Source: CAD feature listing. Evaluate the final solid. Frame: model axes, mm. Round coordinates to 2 decimals unless told otherwise and drop trailing zeros. Order: outer loops, then holes, each group sorted by start corner. A loop starts at its lowest first (then second) coordinate and runs counter-clockwise, first axis right, second up. Notation, with made-up numbers: (-20.75, 45) -> (35.25, 45) arc R22 cw to (35.25, 61) -> close; hole circle Ø10 at (70.5, 63). An arc over 180 degrees is marked (long way). Answer as CSV lines item,"result".
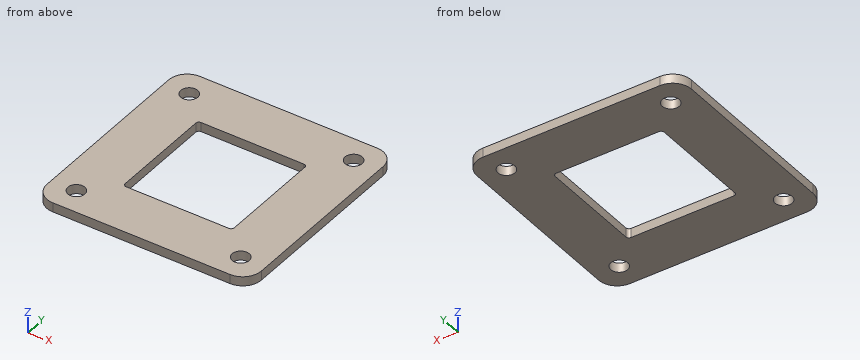
Autodesk Inventor part; units mm, degrees
ref_plane "YZ Plane" through (0, 0, 0) normal (1, 0, 0) x (0, 1, 0)
ref_plane "XZ Plane" through (0, 0, 0) normal (0, 1, 0) x (-1, 0, 0)
ref_plane "XY Plane" through (0, 0, 0) normal (0, 0, 1) x (1, 0, 0)
sketch "Sketch1" plane through (0, 0, 0) normal (0, 0, 1) x (1, 0, 0)
  line L0 (-34.6, -34.6) -> (34.6, -34.6)
  line L1 (34.6, -34.6) -> (34.6, 34.6)
  line L2 (34.6, 34.6) -> (-34.6, 34.6)
  line L3 (-34.6, 34.6) -> (-34.6, -34.6)
  line L4 (-34.6, -34.6) -> (34.6, 34.6) construction
  line L5 (34.6, -34.6) -> (-34.6, 34.6) construction
  line L6 (17.6, -17.6) -> (-17.6, -17.6)
  line L7 (-17.6, -17.6) -> (-17.6, 17.6)
  line L8 (-17.6, 17.6) -> (17.6, 17.6)
  line L9 (17.6, 17.6) -> (17.6, -17.6)
  line L10 (17.6, -17.6) -> (-17.6, 17.6) construction
  line L11 (-17.6, -17.6) -> (17.6, 17.6) construction
  point P0 (0, 0)
  dimension "d172" = 35.2
  dimension "d181" = 17
  dimension "d187" = 17
extrude "Plate5" add sketch "Sketch1" along normal blind 3
sketch "Sketch9" plane through (0, 0, 3) normal (0, 0, 1) x (1, 0, 0)
  circle A0 centre (26.5165, -26.5165) radius 2.75
  line L0 (26.5165, 26.5165) -> (-26.5165, 26.5165) construction
  line L1 (-26.5165, 26.5165) -> (-26.5165, -26.5165) construction
  line L2 (-26.5165, -26.5165) -> (26.5165, -26.5165) construction
  line L3 (26.5165, -26.5165) -> (26.5165, 26.5165) construction
  line L4 (26.5165, 26.5165) -> (-26.5165, -26.5165) construction
  line L5 (-26.5165, 26.5165) -> (26.5165, -26.5165) construction
  circle A1 centre (-26.5165, -26.5165) radius 2.75
  circle A2 centre (26.5165, 26.5165) radius 2.75
  circle A3 centre (-26.5165, 26.5165) radius 2.75
  circle A4 centre (0, 0) radius 37.5 construction
  line L6 (-17.6, -17.6) -> (-17.6, 17.6)
  line L7 (-17.6, 17.6) -> (17.6, 17.6)
  line L8 (17.6, 17.6) -> (17.6, -17.6)
  line L9 (17.6, -17.6) -> (-17.6, -17.6)
  line L10 (34.6, -34.6) -> (-34.6, -34.6)
  line L11 (34.6, 34.6) -> (34.6, -34.6)
  line L12 (-34.6, 34.6) -> (34.6, 34.6)
  line L13 (-34.6, -34.6) -> (-34.6, 34.6)
  line L14 (-15, 15) -> (15, 15) construction
  line L15 (15, 15) -> (15, -15) construction
  line L16 (15, -15) -> (-15, -15) construction
  line L17 (-15, -15) -> (-15, 15) construction
  line L18 (-15, -15) -> (15, 15) construction
  dimension "d188" = 75
  dimension "d174" = 5.5
  dimension "d184" = 30
  dimension "d185" = 30
  dimension "d186" = 16.2868
extrude "Cut2" cut sketch "Sketch9" against normal blind 3 contours A0 | A1 | A2 | A3
fillet "Corner Round1" radius 6 4 edges at (34.6, 34.6, 1.5) (-34.6, 34.6, 1.5) (-34.6, -34.6, 1.5) (34.6, -34.6, 1.5)
fillet "Corner Round2" radius 1 4 edges at (-17.6, 17.6, 1.5) (-17.6, -17.6, 1.5) (17.6, -17.6, 1.5) (17.6, 17.6, 1.5)
properties part number "ANP 1425 FDS Way FLANGE" material "Stainless Steel"
1. Section query D-D on z = 1.45. Return loops of the section in (x, y).
Results below:
outline,"(-34.6, -28.6) arc R6 ccw to (-28.6, -34.6) -> (28.6, -34.6) arc R6 ccw to (34.6, -28.6) -> (34.6, 28.6) arc R6 ccw to (28.6, 34.6) -> (-28.6, 34.6) arc R6 ccw to (-34.6, 28.6) -> close; hole circle Ø5.5 at (-26.52, -26.52); hole circle Ø5.5 at (-26.52, 26.52); hole (-17.6, -16.6) arc R1 ccw to (-16.6, -17.6) -> (16.6, -17.6) arc R1 ccw to (17.6, -16.6) -> (17.6, 16.6) arc R1 ccw to (16.6, 17.6) -> (-16.6, 17.6) arc R1 ccw to (-17.6, 16.6) -> close; hole circle Ø5.5 at (26.52, -26.52); hole circle Ø5.5 at (26.52, 26.52)"
2. Line query: L1, parallel to Y at x = -6, z = 2.8; L2, parallel to X at y = -27, z = 1.85. Output: solid intervals per line, ascending. Write a range as [from, to].
Results below:
L1,"[-34.6, -17.6], [17.6, 34.6]"
L2,"[-34.6, -29.22], [-23.81, 23.81], [29.22, 34.6]"
3. Section query C-C on x = -25. Return loops of the section in (y, z).
Results below:
outline,"(-34.6, 0) -> (-28.81, 0) -> (-28.81, 3) -> (-34.6, 3) -> close; (-24.22, 0) -> (24.22, 0) -> (24.22, 3) -> (-24.22, 3) -> close; (28.81, 0) -> (34.6, 0) -> (34.6, 3) -> (28.81, 3) -> close"
4. Pin query (flat end, axial travel): pin 1 (4.5 mm diameter, centred on x = -26.52, y = 26.52, fed in from -Z). Return the tip coordinate at first contact, or that it passes through.
Results below:
pin 1,"through"
5. Section query A-A on y = 2.5. Return loops of the section in (x, z).
Results below:
outline,"(-34.6, 0) -> (-17.6, 0) -> (-17.6, 3) -> (-34.6, 3) -> close; (17.6, 0) -> (34.6, 0) -> (34.6, 3) -> (17.6, 3) -> close"
